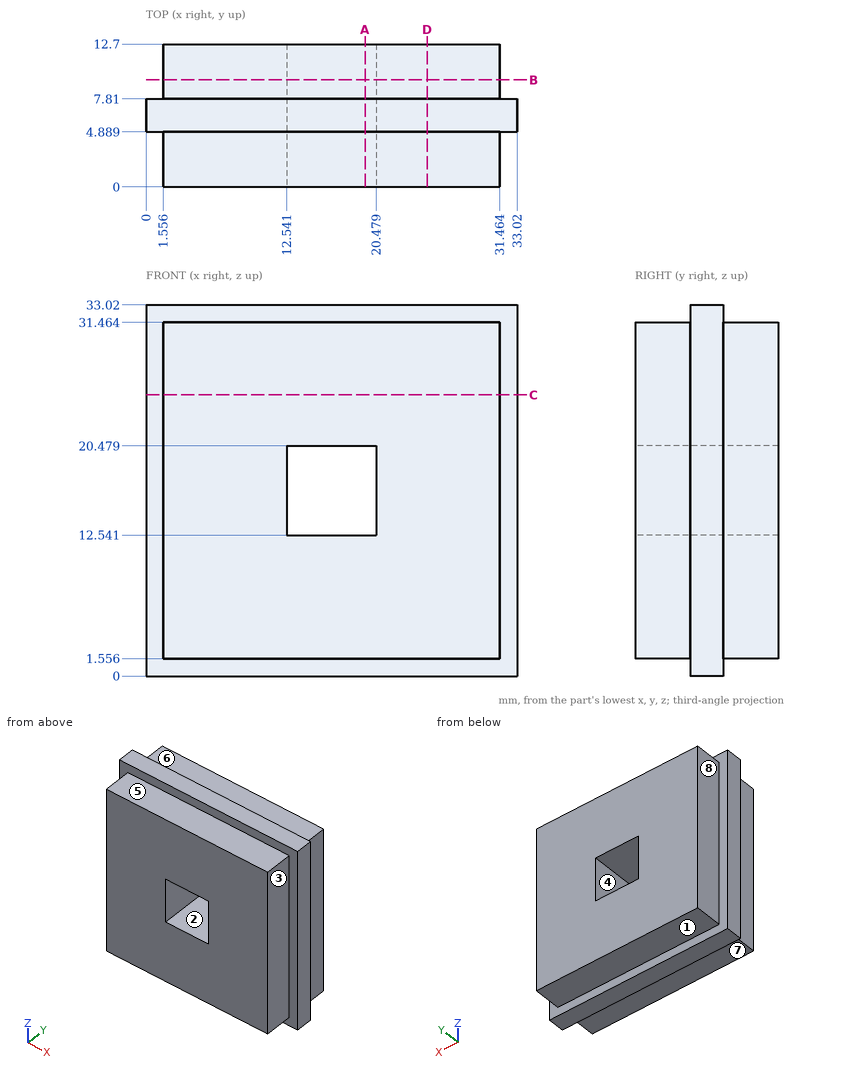
For this review, use the dimensioned drawing (mm, ordinates from the lowest corner) and the shaded views. A direction names the side the tool comes from. Give positions to 0.01 mm unless a question says otherwise; leave off trailing zeros. Order: outer loops, then holes, each group sorted by start corner. A loop starts at its lowest first (then second) coordinate and runs counter-clockwise, first axis right, second up. Notation, with made-up numbers: M 83.25,20 L 122.25,20 A15 cw 122.25,38 Z; hole C -23.75,20 d9. An arc over 180 degrees is marked long. Use one line per item in the form item = value. Start each with the question number.
Item 1: We need section C-C on z = 25. Give the boundary of the cut face in (x, y) (1 decimal).
Item 2: To check wall thickness, follow line 1 along X through (y, z) = (10.75, 14.5) (1 decimal); line 2 along Z through (x, y) = (9, 3) (1 decimal). State the ranges of each line that lie inside material, in increasing order. Write a range as from..to.
Item 3: The part is to be moulded in two halves that separate along X. For the marked faces 1, 2 and 3, say which applies: pulls with the +X half, pulls with the -X half, needs draft (parallel to the pull), parting line crosses it, or undercut.
Item 4: Insertion check: pin 1 Ø2.5 at (y, z) = (7.5, 15) entering from -X; pin 2 Ø1.5 at (x, y) = (25.5, 10.5) entering from -Z; pin 3 Ø1.5 at (y, z) = (9.5, 15) entering from +X; pin 4 Ø2.5 at (x, y) = (11, 11.5) entering from +Z. Each pin has a flat end and moves straight along its axis. Give the tip position at first contact, or say it passes through.
Item 5: We need section B-B on y = 9.5. Give the boundary of the cut face in (x, z) (1 decimal).
Item 6: For the marked faces 4, 5, 6, 7 and 8, list the 3-axis set-ups (+Z, -Z, +X, -X, +Y, -Y) from which the entire face can be reached by the end or side of a thin tool; tool diameter is ignored.
Item 7: We need section A-A on x = 19.5. Give the boundary of the cut face in (y, z) (1 decimal), plus the area to 3 significant figures.
Item 8: We need section D-D on x = 25. Give the boundary of the cut face in (y, z) (1 decimal), plus the area to 3 significant figures.
Completed:
q1.outline = M 0,4.9 L 1.6,4.9 L 1.6,0 L 31.5,0 L 31.5,4.9 L 33,4.9 L 33,7.8 L 31.5,7.8 L 31.5,12.7 L 1.6,12.7 L 1.6,7.8 L 0,7.8 Z
q2.line_1 = 1.6..12.5, 20.5..31.5
q2.line_2 = 1.6..31.5
q3.face_1 = needs draft
q3.face_2 = undercut
q3.face_3 = pulls with the +X half
q4.pin_1 = 0
q4.pin_2 = 1.56
q4.pin_3 = 31.46
q4.pin_4 = 31.46
q5.outline = M 1.6,1.6 L 31.5,1.6 L 31.5,31.5 L 1.6,31.5 Z; hole M 12.5,12.5 L 20.5,12.5 L 20.5,20.5 L 12.5,20.5 Z
q6.face_4 = +Y, -Y
q6.face_5 = +Z, +X, -X, -Y
q6.face_6 = +Z, +X, -X, +Y
q6.face_7 = -Z, +X, -X, -Y
q6.face_8 = +Z, -Z, -X, +Y
q7.outline = M 0,1.6 L 4.9,1.6 L 4.9,0 L 7.8,0 L 7.8,1.6 L 12.7,1.6 L 12.7,12.5 L 0,12.5 Z; M 0,20.5 L 12.7,20.5 L 12.7,31.5 L 7.8,31.5 L 7.8,33 L 4.9,33 L 4.9,31.5 L 0,31.5 Z
q7.area = 288 mm²
q8.outline = M 0,1.6 L 4.9,1.6 L 4.9,0 L 7.8,0 L 7.8,1.6 L 12.7,1.6 L 12.7,31.5 L 7.8,31.5 L 7.8,33 L 4.9,33 L 4.9,31.5 L 0,31.5 Z
q8.area = 389 mm²
